```python
from build123d import *

# Parameters (mm, degrees)
BOSS_EXTRUDE1_DEPTH = 5.5
FILLET1_R           = 2
SKETCH2_R           = 22.114757516
BOSS_EXTRUDE2_DEPTH = 5.2
CUT_EXTRUDE1_DEPTH  = 4.2
SKETCH4_R           = 2.2
CUT_EXTRUDE2_DEPTH  = 4.2


with BuildPart() as part:
    # Sketch1 → Boss-Extrude1 (new body)
    with BuildSketch(Plane(origin=(0, 0, 0), x_dir=(1, 0, 0), z_dir=(0, 1, 0))):
        with BuildLine():
            ThreePointArc((1.5, 0), (-1.060660172, -1.060660172), (0, 1.5))
            Line((0, 1.5), (0, 22.5))
            ThreePointArc((0, 22.5), (-1.060660172, 25.060660172), (1.5, 24))
            Line((1.5, 24), (9.75, 24))
            Line((9.75, 24), (9.75, 28.5))
            Line((9.75, 28.5), (9.75, 34))
            ThreePointArc((9.75, 34), (12, -10.114757516), (14.25, 34))
            Line((14.25, 34), (14.25, 28.5))
            Line((14.25, 28.5), (14.25, 24))
            Line((14.25, 24), (22.5, 24))
            ThreePointArc((22.5, 24), (25.060660172, 25.060660172), (24, 22.5))
            Line((24, 22.5), (24, 1.5))
            ThreePointArc((24, 1.5), (25.060660172, -1.060660172), (22.5, 0))
            Line((22.5, 0), (1.5, 0))
        make_face()
        with BuildLine():
            Line((9.75, 34), (9.75, 28.5))
            Line((9.75, 28.5), (14.25, 28.5))
            Line((14.25, 28.5), (14.25, 34))
            ThreePointArc((14.25, 34), (12, 34.114757516), (9.75, 34))
        make_face()
    extrude(amount=BOSS_EXTRUDE1_DEPTH)

    # Fillet1
    fillet1_edges = [part.edges().sort_by_distance(p)[0] for p in [
        (0, 2.75, -22.5),
        (0, 2.75, -1.5),
        (1.5, 2.75, 0),
        (22.5, 2.75, 0),
        (24, 2.75, -1.5),
        (24, 2.75, -22.5),
        (22.5, 2.75, -24),
        (1.5, 2.75, -24),
    ]]
    fillet(fillet1_edges, radius=FILLET1_R)

    # Sketch2 → Boss-Extrude2 (add)
    with BuildSketch(Plane(origin=(0, 5.5, 0), x_dir=(1, 0, 0), z_dir=(0, 1, 0))):
        with Locations(Location((12, 12, 0), (0, 0, 270))):
            Circle(SKETCH2_R)
    extrude(amount=BOSS_EXTRUDE2_DEPTH)

    # Sketch3 → Cut-Extrude1 (cut)
    with BuildSketch(Plane(origin=(0, 10.7, 0), x_dir=(1, 0, 0), z_dir=(0, 1, 0))):
        Polygon((16.849742261, 12), (14.424871131, 16.2), (9.575128869, 16.2), (7.150257739, 12), (9.575128869, 7.8), (14.424871131, 7.8), align=None)
    extrude(amount=-CUT_EXTRUDE1_DEPTH, mode=Mode.SUBTRACT)

    # Sketch4 → Cut-Extrude2 (cut)
    with BuildSketch(Plane(origin=(0, 6.5, 0), x_dir=(1, 0, 0), z_dir=(0, 1, 0))):
        with Locations(Location((12, 12, 0), (0, 0, 270))):
            Circle(SKETCH4_R)
    extrude(amount=-CUT_EXTRUDE2_DEPTH, mode=Mode.SUBTRACT)


solid = part.part
```
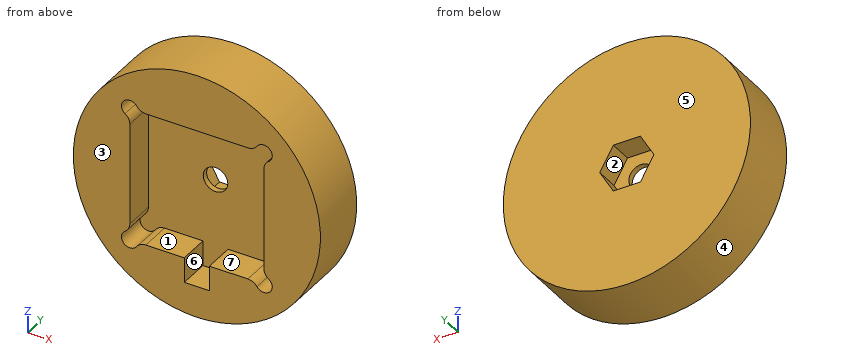
Here's how the part is built. I have some questions about the finished solid (model axes, mm). Face numbers are marked on the shaded views. A direction names the side the tool comes from. Give positions to 0.01 mm unless a question says otherwise; leave off trailing zeros. Loops run counter-clockwise (first coordinate to the right, second up) from the corner with the lowest first, then second, coordinate; pieces in that order, holes last. Notation, with made-up numbers: M -9,25 L 26,25 A7 cw 26,34 Z; hole C 53,-19.5 d11. An arc over 180 degrees is marked long. Use one line per item in the form item = value. Start each with the question number.
Q1. If we section it at A-A (y = 1.5): Write out the boundary of the cut face in (x, z).
Q2. Which directions (+Z, -Z, +X, -X, +Y, -Y) give clear straight access to the entire face, cutting with the end or side of a thin tool? Please do the marked faces 1, 2 and 3.
Q3. If we section it at B-B (y = 9.25): Write out the boundary of the cut face in (x, z).
Q4. If we section it at D-D (x = 16): Write out the boundary of the cut face in (y, z), then the cut area to 3 significant figures.
Q5. I need wall thicknesses on line 1 along Y through (x, z) = (16, -9); line 2 along Z through (x, y) = (10.5, 1); line 3 along Z through (x, y) = (18.5, 4). Which ranges of each line are inside material? Lowest first, please.
Q6. Will these pins go through, and if not, where does the flat tip stop? pin 1 Ø6 at (y, z) = (8.5, 3) entering from +X; pin 2 Ø4 at (x, z) = (7.5, -21) entering from -Y; pin 3 Ø1.5 at (y, z) = (8, 0) entering from -X.
Q7. Thinking about a two-plate mould opening in Z: for the marked faces 4, 5, 6 and 7, which applies, +Z half, -Z half, draft (parallel to the pull), parting line (faces both ways), or undercut?
Taken from the geometry:
q1.outline = C 12,-12 d44.23; hole M -0.86,-22.77 A1.5 ccw long 1.23,-24.86 A2 cw 2.87,-24 L 9.75,-24 L 9.75,-28.5 L 14.25,-28.5 L 14.25,-24 L 21.13,-24 A2 cw 22.77,-24.86 A1.5 ccw long 24.86,-22.77 A2 cw 24,-21.13 L 24,-2.87 A2 cw 24.86,-1.23 A1.5 ccw long 22.77,0.86 A2 cw 21.13,0 L 2.87,0 A2 cw 1.23,0.86 A1.5 ccw long -0.86,-1.23 A2 cw 0,-2.87 L 0,-21.13 A2 cw Z
q2.face_1 = -Y
q2.face_2 = +Y
q2.face_3 = +Z, -Z, +X, -X, -Y
q3.outline = C 12,-12 d44.23; hole M 7.15,-12 L 9.58,-16.2 L 14.42,-16.2 L 16.85,-12 L 14.42,-7.8 L 9.58,-7.8 Z
q4.outline = M 0,-33.75 L 10.7,-33.75 L 10.7,-13.47 L 6.5,-13.47 L 6.5,-10.53 L 10.7,-10.53 L 10.7,9.75 L 0,9.75 L 0,0 L 5.5,0 L 5.5,-24 L 0,-24 Z
q4.area = 321 mm^2
q5.line_1 = 5.5 to 10.7
q5.line_2 = -34.06 to -28.5, 0 to 10.06
q5.line_3 = -33.14 to -24, 0 to 9.14
q6.pin_1 = 30.58
q6.pin_2 = 5.5
q6.pin_3 = -7.04
q7.face_4 = parting line
q7.face_5 = draft
q7.face_6 = undercut
q7.face_7 = undercut
